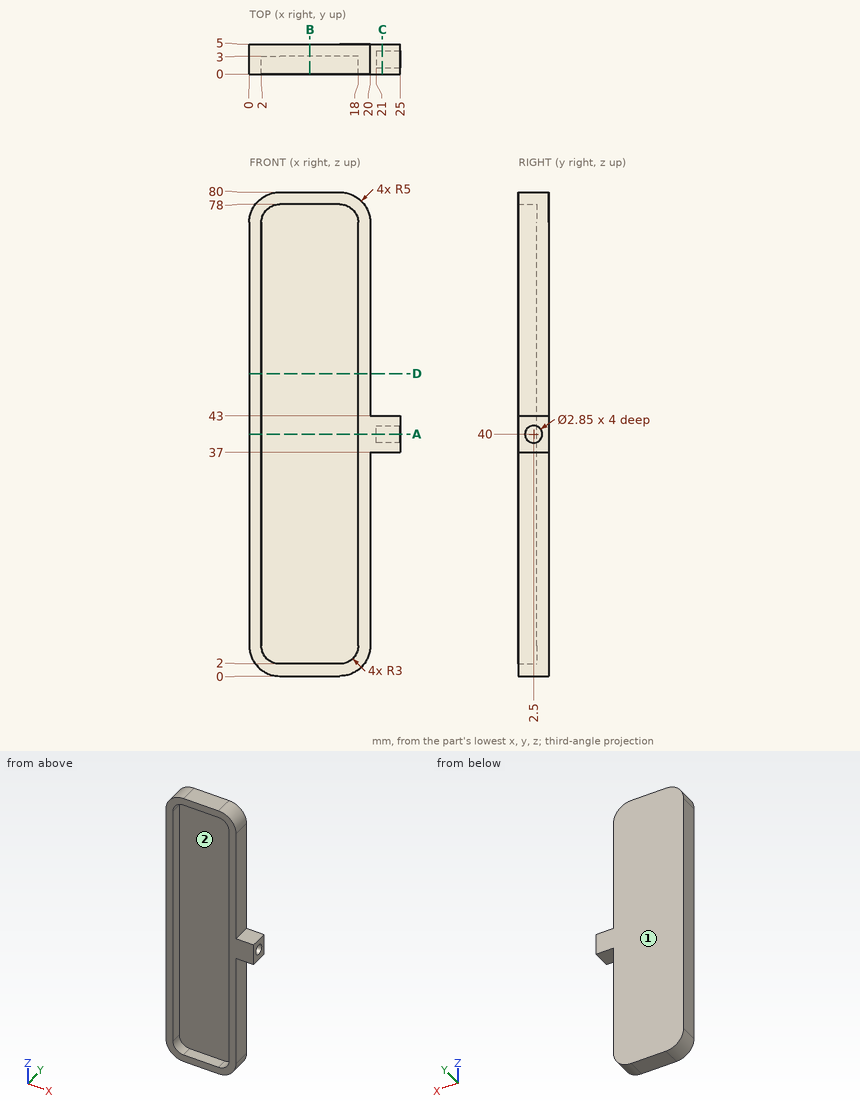
Job drawing, mm, ordinate dimensions from the low corner. One solid piece. Round coordinates to 2 decimals unless told otherwise and drop trailing zeros. Loops run counter-clockwise (first coordinate to the right, second up) from the corner with the lowest first, then second, coordinate; pieces in that order, holes last.
Item 1: Cut at B-B, the plane x = 10. Give the cut face in (y, z).
Item 2: Drop flat-ended pins along their axis: P1, Ø0.9, axis at y = 2, z = 28, coming from the +X side; P2, Ø8, axis at x = 9.5, z = 57, coming from the -Y side; P3, Ø2.5, axis at x = 23.5, y = 2.5, coming from the -Z side. Give the stop position or say it passes through.
Item 3: Drill centre lines: line 1 (X direction, y = 0.45, z = 29); line 2 (Y direction, x = 23.5, z = 40) (3 decimals); line 3 (Z direction, x = 13.75, y = 0.55). Where is each one in solid material? Low to high.
Item 4: Cut at D-D, the plane z = 50. Give the cut face in (x, y).
Item 5: Cut at C-C, the plane x = 22. Give the cut face in (y, z) (3 decimals).
Item 6: Cut at A-A, the plane z = 40. Give the cut face in (x, y) (3 decimals), then the cut area to 3 significant figures.
Item 7: Mould opens along Y. For the marked faces 1 and 2 say: +Y half, -Y half, draft (parallel to the pull), parting line (faces both ways), or undercut.
A:
1. outline: (0, 0) - (5, 0) - (5, 80) - (0, 80) - (0, 78) - (3, 78) - (3, 2) - (0, 2) - close
2. P1: stops at x = 20
2. P2: stops at y = 3
2. P3: stops at z = 37
3. line 1: x = 0 to 2, 18 to 20
3. line 2: y = 0 to 1.075, 3.925 to 5
3. line 3: z = 0 to 2, 78 to 80
4. outline: (0, 0) - (2, 0) - (2, 3) - (18, 3) - (18, 0) - (20, 0) - (20, 5) - (0, 5) - close
5. outline: (0, 37) - (5, 37) - (5, 43) - (0, 43) - close; hole circle Ø2.85 at (2.5, 40)
6. outline: (0, 0) - (2, 0) - (2, 3) - (18, 3) - (18, 0) - (25, 0) - (25, 1.075) - (21, 1.075) - (21, 3.925) - (25, 3.925) - (25, 5) - (0, 5) - close
6. area: 65.6 mm2
7. face 1: +Y half
7. face 2: -Y half
